Autodesk Inventor part; units mm, degrees
ref_plane "YZ Plane" through (0, 0, 0) normal (1, 0, 0) x (0, 1, 0)
ref_plane "XZ Plane" through (0, 0, 0) normal (0, 1, 0) x (-1, 0, 0)
ref_plane "XY Plane" through (0, 0, 0) normal (0, 0, 1) x (1, 0, 0)
sketch "スケッチ1" plane through (0, 0, 0) normal (0, 0, 1) x (1, 0, 0)
  line L0 (-24.75, 20) -> (24.75, 20)
  line L1 (24.75, 20) -> (24.75, -20)
  line L2 (24.75, -20) -> (-24.75, -20)
  line L3 (-24.75, -20) -> (-24.75, 20)
  line L4 (-24.75, 20) -> (24.75, -20) construction
  line L5 (24.75, 20) -> (-24.75, -20) construction
  line L6 (-31, 13.4) -> (31, 13.4)
  line L7 (31, 13.4) -> (31, -13.4)
  line L8 (31, -13.4) -> (-31, -13.4)
  line L9 (-31, -13.4) -> (-31, 13.4)
  line L10 (-31, 13.4) -> (31, -13.4) construction
  line L11 (31, 13.4) -> (-31, -13.4) construction
  line L12 (-19, 5) -> (19, 5)
  line L13 (19, 5) -> (19, -5)
  line L14 (19, -5) -> (-19, -5)
  line L15 (-19, -5) -> (-19, 5)
  line L16 (-19, 5) -> (19, -5) construction
  line L17 (19, 5) -> (-19, -5) construction
  point P0 (0, 0)
  point P1 (-24.75, 13.4)
  point P2 (-24.75, -13.4)
  point P3 (24.75, -13.4)
  point P4 (24.75, 13.4)
  dimension "d0" = 49.5
  dimension "d1" = 40
  dimension "d2" = 62
  dimension "d3" = 26.8
  dimension "d4" = 38
  dimension "d5" = 10
extrude "押し出し1" add sketch "スケッチ1" along normal blind 4
fillet "フィレット1" radius 3 4 edges at (-19, 5, 2) (19, 5, 2) (-19, -5, 2) (19, -5, 2)
fillet "フィレット2" radius 2 8 edges at (24.75, 20, 2) (31, 13.4, 2) (31, -13.4, 2) (24.75, -20, 2) (-24.75, 20, 2) (-31, 13.4, 2) (-31, -13.4, 2) (-24.75, -20, 2)
properties part number "top"
The listing builds one solid part. Answer for the finished solid, in the listing's coordinates (mm). A direction names the side the tool comes from. Round coordinates to 2 decimals unless told otherwise and drop trailing zeros. Loops run counter-clockwise (first coordinate to the right, second up) from the corner with the lowest first, then second, coordinate; pieces in that order, holes last. Notation, with made-up numbers: (72, 75.25) - (122, 75.25) arc R23 ccw to (122, 96.25) - close; hole circle Ø7 at (89.5, 8). An arc over 180 degrees is marked (long way). Return JSON: item names as keys, results as strings. Group by question number.
1. The part is cut by section A-A on x = 4.5. Determine the outline of the cut face in (y, z).
2. Each of these flat-tipped pins is pushed along its axis until it touches: P1, Ø2, axis at x = -27, z = 2.5, coming from the +Y side; P2, Ø2, axis at x = -26, z = 2.5, coming from the -Y side; P3, Ø2, axis at y = -15.5, z = 1, coming from the +X side. Where does it stop, or does it pass through?
3. Which of the six approach directions +Z, -Z, +X, -X, +Y, -Y give full straight-line access (tool end or side, diameter ignored) to faces 1 (the flat face through (0, 20, 2)), 2 (the flat face through (27, -13.4, 2)), 3 (the flat face through (-27, -13.4, 2)), 4 (the flat face through (19, 0, 2)), 5 (the flat face through (24.75, 16, 2))?
4. The part is cut by section D-D on x = 24. Determine the outline of the cut face in (y, z), then the cut area to 3 significant figures.
5. The part is cut by section B-B on y = 0.5. Determine the outline of the cut face in (x, z), then the cut area to 3 significant figures.
6. Consider probe 1 along Y at (x, z) = (0.5, 2.35); probe 2 along X at (y, z) = (-1.5, 1.35); probe 3 along X at (y, z) = (3, 0.25). Determine where each line is inside the solid, lowest interval first.
7. The part is cut by section C-C on z = 3.15. Determine the outline of the cut face in (x, y).
8. The mould has two halves that part along X. Classify faces 6 (the cylindrical face through (-18.14, -4.1, 2.03)), 7 (the flat face through (-27, 13.4, 2)), 8 (the cylindrical face through (30.4, -12.83, 2.03)), 9 (the cylindrical face through (-24.15, 19.43, 2.03)): pulls with the +X half, pulls with the -X half, needs draft (parallel to the pull), parting line crosses it, or undercut.
Resolved:
{
 "1": {"outline": "(-20, 0) - (-5, 0) - (-5, 4) - (-20, 4) - close; (5, 0) - (20, 0) - (20, 4) - (5, 4) - close"},
 "2": {"P1": "stops at y = 13.4", "P2": "stops at y = -13.4", "P3": "stops at x = 24.75"},
 "3": {"face 1": "+Z, -Z, +X, -X, +Y", "face 2": "+Z, -Z, +X, -Y", "face 3": "+Z, -Z, -X, -Y", "face 4": "+Z, -Z", "face 5": "+Z, -Z, +X, +Y"},
 "4": {"outline": "(-19.56, 0) - (19.56, 0) - (19.56, 4) - (-19.56, 4) - close", "area": "156 mm²"},
 "5": {"outline": "(-31, 0) - (-19, 0) - (-19, 4) - (-31, 4) - close; (19, 0) - (31, 0) - (31, 4) - (19, 4) - close", "area": "96.0 mm²"},
 "6": {"probe 1": "y = -20 to -5, 5 to 20", "probe 2": "x = -31 to -19, 19 to 31", "probe 3": "x = -31 to -18.83, 18.83 to 31"},
 "7": {"outline": "(-31, -11.4) arc R2 ccw to (-29, -13.4) - (-24.75, -13.4) - (-24.75, -18) arc R2 ccw to (-22.75, -20) - (22.75, -20) arc R2 ccw to (24.75, -18) - (24.75, -13.4) - (29, -13.4) arc R2 ccw to (31, -11.4) - (31, 11.4) arc R2 ccw to (29, 13.4) - (24.75, 13.4) - (24.75, 18) arc R2 ccw to (22.75, 20) - (-22.75, 20) arc R2 ccw to (-24.75, 18) - (-24.75, 13.4) - (-29, 13.4) arc R2 ccw to (-31, 11.4) - close; hole (-19, -2) arc R3 ccw to (-16, -5) - (16, -5) arc R3 ccw to (19, -2) - (19, 2) arc R3 ccw to (16, 5) - (-16, 5) arc R3 ccw to (-19, 2) - close"},
 "8": {"face 6": "undercut", "face 7": "needs draft", "face 8": "pulls with the +X half", "face 9": "pulls with the -X half"}
}
